```python
from build123d import *

# Parameters (mm, degrees)
SKETCH1_RX          = 12.847459174
SKETCH1_RY          = 12.7
BOSS_EXTRUDE1_DEPTH = 1.5875
SKETCH3_R           = 13.081
CUT_EXTRUDE1_DEPTH  = 118.1481
SKETCH4_R           = 13.081
CUT_EXTRUDE2_DEPTH  = 118.1481
FILLET1_R           = 25.4


with BuildPart() as part:
    # Sketch1 → Boss-Extrude1 (new, symmetric)
    with BuildSketch(Plane.ZY.offset(573.7606)):
        with BuildLine():
            Line((38.1, 225.425), (38.1, 183.869089605))
            ThreePointArc((38.1, 183.869089605), (18.348846559, 164.117936165), (-1.402306881, 183.869089605))
            Line((-1.402306881, 183.869089605), (-1.402306881, 225.425))
            Line((-1.402306881, 225.425), (-139.7, 225.425))
            Line((-139.7, 225.425), (-139.7, 92.075))
            Line((-139.7, 92.075), (-105.5624, 92.075))
            Line((-105.5624, 92.075), (-105.5624, 88.9))
            Line((-105.5624, 88.9), (-139.7, 88.9))
            Line((-139.7, 88.9), (-139.7, -88.9))
            Line((-139.7, -88.9), (-105.5624, -88.9))
            Line((-105.5624, -88.9), (-105.5624, -92.075))
            Line((-105.5624, -92.075), (-139.7, -92.075))
            Line((-139.7, -92.075), (-139.7, -225.425))
            Line((-139.7, -225.425), (-1.402306881, -225.425))
            Line((-1.402306881, -225.425), (-1.402306881, -183.869089605))
            ThreePointArc((-1.402306881, -183.869089605), (18.348846559, -164.117936165), (38.1, -183.869089605))
            Line((38.1, -183.869089605), (38.1, -225.425))
            Line((38.1, -225.425), (63.5, -225.425))
            Line((63.5, -225.425), (63.5, -60.325))
            Line((63.5, -60.325), (124.46, -60.325))
            Line((124.46, -60.325), (124.46, -280.035))
            Line((124.46, -280.035), (207.01, -280.035))
            Line((207.01, -280.035), (207.01, 280.035))
            Line((207.01, 280.035), (124.46, 280.035))
            Line((124.46, 280.035), (124.46, 60.325))
            Line((124.46, 60.325), (63.5, 60.325))
            Line((63.5, 60.325), (63.5, 225.425))
            Line((63.5, 225.425), (38.1, 225.425))
        make_face()
        with Locations(Location((-40.479630886, 184.911482002), (0, 0, 94.708027414))):
            Ellipse(SKETCH1_RX, SKETCH1_RY, mode=Mode.SUBTRACT)
        with Locations(Location((-40.479630886, -184.911482002), (0, 0, -94.708027414))):
            Ellipse(SKETCH1_RX, SKETCH1_RY, mode=Mode.SUBTRACT)
    extrude(amount=BOSS_EXTRUDE1_DEPTH, both=True)

    # Sketch3 → Cut-Extrude1 (cut)
    with BuildSketch(Plane(origin=(-457.2, 191.578892686, 65.734499214), x_dir=(0, 0, 1), z_dir=(-1, 0, 0))):
        Circle(SKETCH3_R)
    cut_extrude1 = extrude(amount=CUT_EXTRUDE1_DEPTH, mode=Mode.SUBTRACT)

    # Sketch4 → Cut-Extrude2 (cut)
    with BuildSketch(Plane(origin=(-457.2, 243.726115798, 209.007817696), x_dir=(0, 0, -1), z_dir=(1, 0, 0))):
        Circle(SKETCH4_R)
    cut_extrude2 = extrude(amount=-CUT_EXTRUDE2_DEPTH, mode=Mode.SUBTRACT)

    # Mirror1: Cut-Extrude1, Cut-Extrude2 across plane
    add(cut_extrude1.mirror(Plane.ZX), mode=Mode.SUBTRACT)
    add(cut_extrude2.mirror(Plane.ZX), mode=Mode.SUBTRACT)

    # Fillet1
    fillet1_edges = [part.edges().sort_by_distance(p)[0] for p in [
        (-573.7606, 60.325, 63.5),
        (-573.7606, 60.325, 124.46),
        (-573.7606, -60.325, 124.46),
        (-573.7606, -60.325, 63.5),
    ]]
    fillet(fillet1_edges, radius=FILLET1_R)


solid = part.part
```
Check sheet for the modelled part. Datum: model origin and axes. Units: mm. A direction names the side the tool comes from. Round coordinates to 2 decimals unless told otherwise and drop trailing zeros. Write each loop counter-clockwise with the first axis right and the second up, starting at its lowest first coordinate (ties: lowest second). Pieces come first, ordered by that corner, then holes. Notation, with made-up numbers: (18.5, 46.5) -> (47.5, 46.5) arc R18 ccw to (47.5, 56.5) -> close; hole circle Ø8 at (23, 26.25). An arc over 180 degrees is marked (long way). Put each result on its own line as item: value.
(1) Sectioned sample at B-B (y = -99). Enter the section's corners in (x, z), plus the area to 3 significant figures.
Values found:
outline: (-575.35, -139.7) -> (-572.17, -139.7) -> (-572.17, 63.5) -> (-575.35, 63.5) -> close; (-575.35, 124.46) -> (-572.17, 124.46) -> (-572.17, 207.01) -> (-575.35, 207.01) -> close
area: 907 mm^2
(2) Go/stop test with flat-tipped pins: pin 1 Ø1 at (x, z) = (-574, 94.5) entering from -Y (3 decimals); pin 2 Ø1.6 at (x, y) = (-574.5, -90) entering from -Z; pin 3 Ø1 at (x, z) = (-574, 47) entering from +Y (3 decimals). Record where each tip stops, or that it passes through.
Values found:
pin 1: stops at y = -60.325
pin 2: stops at z = -105.56
pin 3: stops at y = 225.425
(3) Sectioned sample at D-D (x = -574.85). Count the separate pieces of the cut face and the enclosed holes in it, plus the area to 3 significant figures.
Values found:
separate pieces: 1
enclosed holes: 2
area: 139,000 mm^2
(4) Tool access check on faces 1 (the face through (-573.738, 67.568, 116.822)), 2 (the face through (-573.738, 191.835, 52.656)), 3 (the face through (-573.74, -243.47, 195.93)), 4 (the face through (-572.173, 4, 31)), 5 (the face through (-573.738, -67.568, 71.138)). Record the directions out of +Z, -Z, +X, -X, +Y, -Y that give a thin tool (end or side, any length) a straight path to the whole face; none if there is none.
Values found:
face 1: +X, -X, +Y
face 2: +X, -X
face 3: +Z, +X, -X
face 4: +Z, -Z, +X, +Y, -Y
face 5: +X, -X, -Y
(5) Sectioned sample at C-C (z = -8.5). Enter the section's corners in (x, y) (3 decimals), plus the area to 3 significant figures.
Values found:
outline: (-575.348, -225.425) -> (-572.173, -225.425) -> (-572.173, 225.425) -> (-575.348, 225.425) -> close
area: 1,430 mm^2
(6) Sectioned sample at A-A (y = -218). Enter the section's corners in (x, z).
Values found:
outline: (-575.35, -139.7) -> (-572.17, -139.7) -> (-572.17, -1.4) -> (-575.35, -1.4) -> close; (-575.35, 38.1) -> (-572.17, 38.1) -> (-572.17, 63.5) -> (-575.35, 63.5) -> close; (-575.35, 124.46) -> (-572.17, 124.46) -> (-572.17, 207.01) -> (-575.35, 207.01) -> close
(7) Mould release check, pull along Z, two halves, no side actions. Record for faces 6 (the face through (-573.74, 243.47, 195.93)), 7 (the face through (-575.348, 4, 31)), 8 (the face through (-573.738, -67.963, 117.217)): released by +Z, released by -Z, zero draft, split by the parting line, or undercut.
Values found:
face 6: released by +Z
face 7: zero draft
face 8: undercut
(8) Material ranges on line 1 (Y direction, x = -574.35, z = -119.5) (3 decimals); line 2 (Z direction, x = -573.4, y = 177); line 3 (Z direction, x = -574.5, y = 88.5), recorded low to high.
Values found:
line 1: y = -225.425 to -92.075, -88.9 to 88.9, 92.075 to 225.425
line 2: z = -139.7 to -50.47, -30.46 to -0.17, 36.87 to 63.5, 124.46 to 207.01
line 3: z = -139.7 to 63.5, 124.46 to 207.01
